Job drawing, mm, ordinate dimensions from the low corner. One solid piece. Round coordinates to 2 decimals unless told otherwise and drop trailing zeros. Loops run counter-clockwise (first coordinate to the right, second up) from the corner with the lowest first, then second, coordinate; pieces in that order, holes last. Notation, with made-up numbers: (34.25, 48.5) - (78.25, 48.5) arc R20 cw to (78.25, 80.5) - close; hole circle Ø10 at (-21, 70.25). An arc over 180 degrees is marked (long way). One line per question, with ' | ' between items. Start each with the question number.
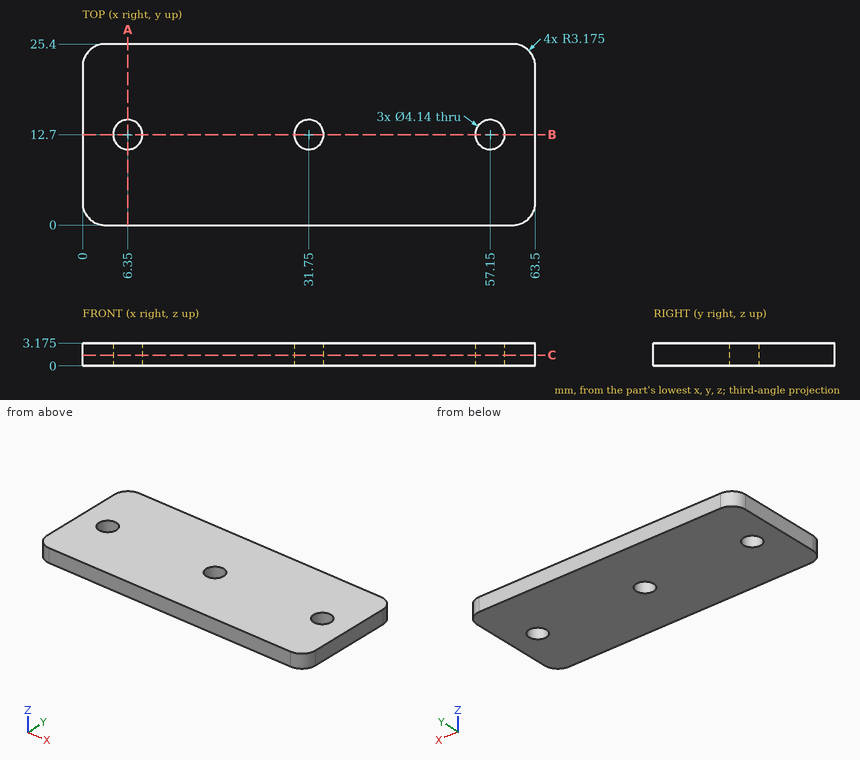
1) Saw through at C-C on z = 1.5. State how many separate pieces and enclosed holes the cut face has, and give its area (3 significant figures).
2) Saw through at B-B on y = 12.7. Write the cut outline in (x, z) (1 decimal).
3) Drop a flat-ended pin along its axis: pin 1 (3.5 mm diameter, centred on x = 31.75, y = 12.7, fed in from +Z). Give the stop position or say it passes through.
4) Wall check: line 1 (Y direction, x = 57.15, z = 1.1); line 2 (X direction, y = 13.25, z = 0.35); line 3 (X direction, y = 23.75, z = 1.5). Give the ranges that are in metal, low to high. Write a range as [from, to].
5) Saw through at A-A on x = 6.35. Write the cut outline in (y, z) (1 decimal).
Answer key:
1) separate pieces: 1 | enclosed holes: 3 | area: 1,560 mm²
2) outline: (0, 0) - (4.3, 0) - (4.3, 3.2) - (0, 3.2) - close; (8.4, 0) - (29.7, 0) - (29.7, 3.2) - (8.4, 3.2) - close; (33.8, 0) - (55.1, 0) - (55.1, 3.2) - (33.8, 3.2) - close; (59.2, 0) - (63.5, 0) - (63.5, 3.2) - (59.2, 3.2) - close
3) pin 1: through
4) line 1: [0, 10.63], [14.77, 25.4] | line 2: [0, 4.35], [8.35, 29.75], [33.75, 55.15], [59.15, 63.5] | line 3: [0.39, 63.11]
5) outline: (0, 0) - (10.6, 0) - (10.6, 3.2) - (0, 3.2) - close; (14.8, 0) - (25.4, 0) - (25.4, 3.2) - (14.8, 3.2) - close
